Could you check a few things on this model? Use its own coordinates, in mm. A direction names the side the tool comes from. Give positions to 0.01 mm unless a question says otherwise; leave off trailing zeros. Loops run counter-clockwise (first coordinate to the right, second up) from the corner with the lowest first, then second, coordinate; pieces in that order, holes last.
1. Imagine slicing it at C-C (z = 0). List the corners of the cut face in (x, y) for me.
2. Imagine slicing it at B-B (x = -7). List the corners of the cut face in (y, z) for me.
3. Thinking about a two-plate mould opening in Z: for faces 1 (the cylindrical face through (-53.766, 14.79, -2.493)), 2 (the flat face through (-16.47, 24.2, 12.93)), 3 (the cylindrical face through (-18.221, 24.463, 4.504)), 4 (the flat face through (46, 15, -3)), which applies, +Z half, -Z half, draft (parallel to the pull), parting line (faces both ways), or undercut?
4. I need wall thicknesses on line 1 along X through (y, z) = (2.5, 5); line 2 along X through (y, z) = (25, 6.5); line 3 along X through (y, z) = (6, 10). Which ranges of each line are inside material? Lowest first, please.
5. For P1, Ø3, axis at x = -20.5, y = 14, coming from the +Z side; P2, Ø4.5, axis at y = 9.5, z = 12, coming from the -X side; P3, Ø2, axis at x = 32, y = 20, coming from the +Z side; P4, Ø14, axis at x = 137.46, z = 0, coming from the -Y side, each with a flat end and sliding along its axis, tell me the tip position at first contact or that it passes through.
6. Imagine slicing it at A-A (y = 7). List the corners of the cut face in (x, z) for me.
7. For faces 5 (the flat face through (-14.267, 22.159, 7.353)), 6 (the flat face through (14.198, 10, 13)), 7 (the flat face through (-25, 18, 3)), 8 (the flat face through (-3, 4.8, 18)), 9 (the flat face through (56, 30, 0)), which set-ups out of +Z, -Z, +X, -X, +Y, -Y let a thin tool reach every point of the face, with its end or its side?
8. Imagine slicing it at D-D (x = 84.5). List the corners of the cut face in (y, z) for me, plus the area to 3 significant figures.
```python
from build123d import *

# Parameters (mm, degrees)
SKETCH1_R           = 11.5
BOSS_EXTRUDE1_DEPTH = 30
CUT_EXTRUDE1_DEPTH  = 10
BOSS_EXTRUDE2_DEPTH = 15
SKETCH4_W           = 34
SKETCH4_H           = 2.123618691
BOSS_EXTRUDE3_DEPTH = 15
FILLET1_R           = 5
SKETCH5_R           = 10.25
CUT_EXTRUDE2_DEPTH  = 15


with BuildPart() as part:
    # Sketch1 → Boss-Extrude1 (new body)
    with BuildSketch(Plane(origin=(0, 0, 0), x_dir=(1, 0, 0), z_dir=(0, 1, 0))):
        with BuildLine():
            Line((-28.353157483, 3), (123.274320599, 3))
            ThreePointArc((123.274320599, 3), (151.960581558, 0), (123.274320599, -3))
            Line((123.274320599, -3), (-28.353157483, -3))
            ThreePointArc((-28.353157483, -3), (-57.039418442, 0), (-28.353157483, 3))
        make_face()
        with Locations(Location((-42.539418442, 0, 0), (0, 0, 270))):
            Circle(SKETCH1_R, mode=Mode.SUBTRACT)
        with Locations(Location((137.460581558, 0, 0), (0, 0, 270))):
            Circle(SKETCH1_R, mode=Mode.SUBTRACT)
    extrude(amount=BOSS_EXTRUDE1_DEPTH)

    # Sketch2 → Cut-Extrude1 (cut)
    with BuildSketch(Plane.XY.offset(3)):
        Polygon((6.198144817, 24.623618691), (-11.801855183, 24.623618691), (-16.801855183, 19.623618691), (-16.801855183, 5.123618691), (11.198144817, 5.123618691), (11.198144817, 19.623618691), align=None)
    extrude(amount=-CUT_EXTRUDE1_DEPTH, mode=Mode.SUBTRACT)

    # Sketch3 → Boss-Extrude2 (add)
    with BuildSketch(Plane.XY.offset(3)):
        Polygon((-13.044495871, 27.623618691), (7.440785504, 27.623618691), (14.198144817, 20.866259379), (14.198144817, 2.123618691), (-19.801855183, 2.123618691), (-19.801855183, 20.866259379), align=None)
        Polygon((-11.801855183, 24.623618691), (-16.801855183, 19.623618691), (-16.801855183, 5.123618691), (11.198144817, 5.123618691), (11.198144817, 19.623618691), (6.198144817, 24.623618691), align=None, mode=Mode.SUBTRACT)
    extrude(amount=BOSS_EXTRUDE2_DEPTH)

    # Sketch4 → Boss-Extrude3 (add)
    with BuildSketch(Plane.XY.offset(3)):
        with Locations((-2.801855183, 1.061809346)):
            Rectangle(SKETCH4_W, SKETCH4_H)
    extrude(amount=BOSS_EXTRUDE3_DEPTH)

    # Fillet1
    # the kernel refuses this fillet: 5 mm, written as the material it adds along each edge
    with BuildSketch(Plane(origin=(-28.640689948, 12.027424614, 3), x_dir=(-0.7071067811865481, 0.7071067811865469, 0), z_dir=(0.707106781186547, 0.7071067811865481, 0))) as fillet1_piece_1_section:
        with BuildLine():
            CenterArc((FILLET1_R, FILLET1_R), FILLET1_R, 180, 90)
            Line((0, FILLET1_R), (0, 0))
            Line((0, 0), (FILLET1_R, 0))
        make_face()
    fillet1_piece_1 = extrude(amount=34.556349186, mode=Mode.PRIVATE)
    fillet1_piece_1 = split(fillet1_piece_1, bisect_by=Plane(origin=(-28.640689948, 27.623618691, 3), z_dir=(0, -1, 0)), keep=Keep.TOP, mode=Mode.PRIVATE)
    fillet1_piece_1 = split(fillet1_piece_1, bisect_by=Plane(origin=(-19.801855183, 12.027424614, 3), z_dir=(1, 0, 0)), keep=Keep.TOP, mode=Mode.PRIVATE)
    add(fillet1_piece_1)
    with BuildSketch(Plane(origin=(-28.640689948, 12.027424614, 3), x_dir=(-0.7071067811865481, 0.7071067811865469, 0), z_dir=(0.707106781186547, 0.7071067811865481, 0))) as fillet1_piece_2_section:
        with BuildLine():
            CenterArc((FILLET1_R, FILLET1_R), FILLET1_R, 180, 90)
            Line((0, FILLET1_R), (0, 0))
            Line((0, 0), (FILLET1_R, 0))
        make_face()
    fillet1_piece_2 = extrude(amount=34.556349186, mode=Mode.PRIVATE)
    fillet1_piece_2 = split(fillet1_piece_2, bisect_by=Plane(origin=(-28.640689948, 27.623618691, 3), z_dir=(0, 1, 0)), keep=Keep.TOP, mode=Mode.PRIVATE)
    fillet1_piece_2 = split(fillet1_piece_2, bisect_by=Plane(origin=(-19.801855183, 12.027424614, 3), z_dir=(-1, 0, 0)), keep=Keep.TOP, mode=Mode.PRIVATE)
    add(fillet1_piece_2)
    with BuildSketch(Plane(origin=(-19.801855183, 0, 3), x_dir=(-1, 0, 0), z_dir=(0, 1, 0))) as fillet1_piece_3_section:
        with BuildLine():
            CenterArc((FILLET1_R, FILLET1_R), FILLET1_R, 180, 90)
            Line((0, FILLET1_R), (0, 0))
            Line((0, 0), (FILLET1_R, 0))
        make_face()
    fillet1_piece_3 = extrude(amount=33.366259379, mode=Mode.PRIVATE)
    fillet1_piece_3 = split(fillet1_piece_3, bisect_by=Plane(origin=(-30.234984873, 10.433129689, 3), z_dir=(0.7071067811865481, -0.707106781186547, 0)), keep=Keep.TOP, mode=Mode.PRIVATE)
    add(fillet1_piece_3)
    with BuildSketch(Plane(origin=(14.198144817, 33.366259379, 3), x_dir=(1, 0, 0), z_dir=(0, -1, 0))) as fillet1_piece_4_section:
        with BuildLine():
            CenterArc((FILLET1_R, FILLET1_R), FILLET1_R, 180, 90)
            Line((0, FILLET1_R), (0, 0))
            Line((0, 0), (FILLET1_R, 0))
        make_face()
    fillet1_piece_4 = extrude(amount=33.366259379, mode=Mode.PRIVATE)
    fillet1_piece_4 = split(fillet1_piece_4, bisect_by=Plane(origin=(7.948144817, 27.116259379, 3), z_dir=(-0.7071067811865476, -0.7071067811865476, 0)), keep=Keep.TOP, mode=Mode.PRIVATE)
    add(fillet1_piece_4)
    with BuildSketch(Plane(origin=(-1.398049261, 36.462453456, 3), x_dir=(0.7071067811865475, 0.7071067811865475, 0), z_dir=(0.7071067811865476, -0.7071067811865476, 0))) as fillet1_piece_5_section:
        with BuildLine():
            CenterArc((FILLET1_R, FILLET1_R), FILLET1_R, 180, 90)
            Line((0, FILLET1_R), (0, 0))
            Line((0, 0), (FILLET1_R, 0))
        make_face()
    fillet1_piece_5 = extrude(amount=34.556349186, mode=Mode.PRIVATE)
    fillet1_piece_5 = split(fillet1_piece_5, bisect_by=Plane(origin=(14.198144817, 36.462453456, 3), z_dir=(-1, 0, 0)), keep=Keep.TOP, mode=Mode.PRIVATE)
    fillet1_piece_5 = split(fillet1_piece_5, bisect_by=Plane(origin=(-1.398049261, 27.623618691, 3), z_dir=(0, -1, 0)), keep=Keep.TOP, mode=Mode.PRIVATE)
    add(fillet1_piece_5)
    with BuildSketch(Plane(origin=(-1.398049261, 36.462453456, 3), x_dir=(0.7071067811865475, 0.7071067811865475, 0), z_dir=(0.7071067811865476, -0.7071067811865476, 0))) as fillet1_piece_6_section:
        with BuildLine():
            CenterArc((FILLET1_R, FILLET1_R), FILLET1_R, 180, 90)
            Line((0, FILLET1_R), (0, 0))
            Line((0, 0), (FILLET1_R, 0))
        make_face()
    fillet1_piece_6 = extrude(amount=34.556349186, mode=Mode.PRIVATE)
    fillet1_piece_6 = split(fillet1_piece_6, bisect_by=Plane(origin=(14.198144817, 36.462453456, 3), z_dir=(1, 0, 0)), keep=Keep.TOP, mode=Mode.PRIVATE)
    fillet1_piece_6 = split(fillet1_piece_6, bisect_by=Plane(origin=(-1.398049261, 27.623618691, 3), z_dir=(0, 1, 0)), keep=Keep.TOP, mode=Mode.PRIVATE)
    add(fillet1_piece_6)
    with BuildSketch(Plane(origin=(-23.685403069, 27.623618691, 3), x_dir=(0, 1, 0), z_dir=(1, 0, 0))) as fillet1_piece_7_section:
        with BuildLine():
            CenterArc((5, 4.256362879), FILLET1_R, 180, 58.350352686)
            Line((0, 4.256362879), (0, 0))
            Line((0, 0), (2.376381309, 0))
        make_face()
    fillet1_piece_7 = extrude(amount=41.767095772, mode=Mode.PRIVATE)
    fillet1_piece_7 = split(fillet1_piece_7, bisect_by=Plane(origin=(-8.122308783, 43.186712978, 3), z_dir=(-0.7071067811865476, -0.7071067811865476, 0)), keep=Keep.TOP, mode=Mode.PRIVATE)
    fillet1_piece_7 = split(fillet1_piece_7, bisect_by=Plane(origin=(-18.36494947, 22.303165092, 3), z_dir=(0.7071067811865481, -0.707106781186547, 0)), keep=Keep.TOP, mode=Mode.PRIVATE)
    add(fillet1_piece_7)
    with BuildSketch(Plane(origin=(-19.801855183, 0, 3), x_dir=(-1, 0, 0), z_dir=(0, 1, 0))) as fillet1_piece_8a_section:
        with BuildLine():
            CenterArc((FILLET1_R, FILLET1_R), FILLET1_R, 180, 90)
            Line((0, FILLET1_R), (0, 0))
            Line((0, 0), (FILLET1_R, 0))
        make_face()
    fillet1_piece_8a = extrude(amount=33.366259379, mode=Mode.PRIVATE)
    fillet1_piece_8a = split(fillet1_piece_8a, bisect_by=Plane(origin=(-30.234984873, 10.433129689, 3), z_dir=(-0.7071067811865481, 0.707106781186547, 0)), keep=Keep.TOP, mode=Mode.PRIVATE)
    fillet1_piece_8a = split(fillet1_piece_8a, bisect_by=Plane(origin=(-19.801855183, 30, 3), z_dir=(0, -1, 0)), keep=Keep.TOP, mode=Mode.PRIVATE)
    with BuildSketch(Plane(origin=(-28.640689948, 12.027424614, 3), x_dir=(-0.7071067811865481, 0.7071067811865469, 0), z_dir=(0.707106781186547, 0.7071067811865481, 0))) as fillet1_piece_8b_section:
        with BuildLine():
            CenterArc((FILLET1_R, FILLET1_R), FILLET1_R, 180, 90)
            Line((0, FILLET1_R), (0, 0))
            Line((0, 0), (FILLET1_R, 0))
        make_face()
    fillet1_piece_8b = extrude(amount=34.556349186, mode=Mode.PRIVATE)
    fillet1_piece_8b = split(fillet1_piece_8b, bisect_by=Plane(origin=(-19.801855183, 12.027424614, 3), z_dir=(-1, 0, 0)), keep=Keep.TOP, mode=Mode.PRIVATE)
    fillet1_piece_8b = fillet1_piece_8b - Plane(origin=(-42.539418442, 12.027424614, 0), x_dir=(0.9783628247662832, 0, 0.20689655172413826), z_dir=(0, -1, 0)) * Cylinder(14.5, 90, mode=Mode.PRIVATE)
    fillet1_piece_8 = fillet1_piece_8a & fillet1_piece_8b
    add(fillet1_piece_8)
    with BuildSketch(Plane(origin=(-28.640689948, 12.027424614, 3), x_dir=(-0.7071067811865481, 0.7071067811865469, 0), z_dir=(0.707106781186547, 0.7071067811865481, 0))) as fillet1_piece_9a_section:
        with BuildLine():
            CenterArc((FILLET1_R, FILLET1_R), FILLET1_R, 180, 90)
            Line((0, FILLET1_R), (0, 0))
            Line((0, 0), (FILLET1_R, 0))
        make_face()
    fillet1_piece_9a = extrude(amount=34.556349186, mode=Mode.PRIVATE)
    fillet1_piece_9a = split(fillet1_piece_9a, bisect_by=Plane(origin=(-28.640689948, 27.623618691, 3), z_dir=(0, 1, 0)), keep=Keep.TOP, mode=Mode.PRIVATE)
    fillet1_piece_9a = split(fillet1_piece_9a, bisect_by=Plane(origin=(-28.640689948, 30, 3), z_dir=(0, -1, 0)), keep=Keep.TOP, mode=Mode.PRIVATE)
    with BuildSketch(Plane(origin=(-23.685403069, 27.623618691, 3), x_dir=(0, 1, 0), z_dir=(1, 0, 0))) as fillet1_piece_9b_section:
        with BuildLine():
            CenterArc((5, 4.256362879), FILLET1_R, 180, 58.350352686)
            Line((0, 4.256362879), (0, 0))
            Line((0, 0), (2.376381309, 0))
        make_face()
    fillet1_piece_9b = extrude(amount=41.767095772, mode=Mode.PRIVATE)
    fillet1_piece_9b = split(fillet1_piece_9b, bisect_by=Plane(origin=(-18.36494947, 22.303165092, 3), z_dir=(-0.7071067811865481, 0.707106781186547, 0)), keep=Keep.TOP, mode=Mode.PRIVATE)
    fillet1_piece_9 = fillet1_piece_9a & fillet1_piece_9b
    add(fillet1_piece_9)
    with BuildSketch(Plane(origin=(-1.398049261, 36.462453456, 3), x_dir=(0.7071067811865475, 0.7071067811865475, 0), z_dir=(0.7071067811865476, -0.7071067811865476, 0))) as fillet1_piece_10a_section:
        with BuildLine():
            CenterArc((FILLET1_R, FILLET1_R), FILLET1_R, 180, 90)
            Line((0, FILLET1_R), (0, 0))
            Line((0, 0), (FILLET1_R, 0))
        make_face()
    fillet1_piece_10a = extrude(amount=34.556349186, mode=Mode.PRIVATE)
    fillet1_piece_10a = split(fillet1_piece_10a, bisect_by=Plane(origin=(14.198144817, 36.462453456, 3), z_dir=(1, 0, 0)), keep=Keep.TOP, mode=Mode.PRIVATE)
    with BuildSketch(Plane(origin=(14.198144817, 33.366259379, 3), x_dir=(1, 0, 0), z_dir=(0, -1, 0))) as fillet1_piece_10b_section:
        with BuildLine():
            CenterArc((FILLET1_R, FILLET1_R), FILLET1_R, 180, 90)
            Line((0, FILLET1_R), (0, 0))
            Line((0, 0), (FILLET1_R, 0))
        make_face()
    fillet1_piece_10b = extrude(amount=33.366259379, mode=Mode.PRIVATE)
    fillet1_piece_10b = split(fillet1_piece_10b, bisect_by=Plane(origin=(7.948144817, 27.116259379, 3), z_dir=(0.7071067811865476, 0.7071067811865476, 0)), keep=Keep.TOP, mode=Mode.PRIVATE)
    fillet1_piece_10b = split(fillet1_piece_10b, bisect_by=Plane(origin=(14.198144817, 30, 3), z_dir=(0, -1, 0)), keep=Keep.TOP, mode=Mode.PRIVATE)
    fillet1_piece_10 = fillet1_piece_10a & fillet1_piece_10b
    add(fillet1_piece_10)
    with BuildSketch(Plane(origin=(-23.685403069, 27.623618691, 3), x_dir=(0, 1, 0), z_dir=(1, 0, 0))) as fillet1_piece_11a_section:
        with BuildLine():
            CenterArc((5, 4.256362879), FILLET1_R, 180, 58.350352686)
            Line((0, 4.256362879), (0, 0))
            Line((0, 0), (2.376381309, 0))
        make_face()
    fillet1_piece_11a = extrude(amount=41.767095772, mode=Mode.PRIVATE)
    fillet1_piece_11a = split(fillet1_piece_11a, bisect_by=Plane(origin=(-8.122308783, 43.186712978, 3), z_dir=(0.7071067811865476, 0.7071067811865476, 0)), keep=Keep.TOP, mode=Mode.PRIVATE)
    with BuildSketch(Plane(origin=(-1.398049261, 36.462453456, 3), x_dir=(0.7071067811865475, 0.7071067811865475, 0), z_dir=(0.7071067811865476, -0.7071067811865476, 0))) as fillet1_piece_11b_section:
        with BuildLine():
            CenterArc((FILLET1_R, FILLET1_R), FILLET1_R, 180, 90)
            Line((0, FILLET1_R), (0, 0))
            Line((0, 0), (FILLET1_R, 0))
        make_face()
    fillet1_piece_11b = extrude(amount=34.556349186, mode=Mode.PRIVATE)
    fillet1_piece_11b = split(fillet1_piece_11b, bisect_by=Plane(origin=(-1.398049261, 27.623618691, 3), z_dir=(0, 1, 0)), keep=Keep.TOP, mode=Mode.PRIVATE)
    fillet1_piece_11b = split(fillet1_piece_11b, bisect_by=Plane(origin=(-1.398049261, 30, 3), z_dir=(0, -1, 0)), keep=Keep.TOP, mode=Mode.PRIVATE)
    fillet1_piece_11 = fillet1_piece_11a & fillet1_piece_11b
    add(fillet1_piece_11)

    # Sketch5 → Cut-Extrude2 (cut)
    with BuildSketch(Plane(origin=(0, 0, -3), x_dir=(-1, 0, 0), z_dir=(0, 0, -1))):
        with Locations((-103.805830626, 15.139955724)):
            Circle(SKETCH5_R)
    extrude(amount=-CUT_EXTRUDE2_DEPTH, mode=Mode.SUBTRACT)


solid = part.part
```
Derived:
1. outline: (-57.04, 0) - (-54.04, 0) - (-54.04, 30) - (-57.04, 30) - close; (-31.04, 0) - (125.96, 0) - (125.96, 30) - (-31.04, 30) - close; (148.96, 0) - (151.96, 0) - (151.96, 30) - (148.96, 30) - close; hole (-16.8, 5.12) - (11.2, 5.12) - (11.2, 19.62) - (6.2, 24.62) - (-11.8, 24.62) - (-16.8, 19.62) - close; hole circle Ø20.5 at (103.81, 15.14)
2. outline: (0, -3) - (5.12, -3) - (5.12, 18) - (0, 18) - close; (24.62, -3) - (30, -3) - (30, 3) arc R5 cw to (27.62, 7.26) - (27.62, 18) - (24.62, 18) - close
3. face 1: undercut
3. face 2: draft
3. face 3: +Z half
3. face 4: -Z half
4. line 1: x = -56.15 to -52.9, -32.18 to -28.93, -20.8 to 15.2, 123.85 to 127.1, 147.82 to 151.07
4. line 2: x = -55.5 to -52.03, -33.05 to -29.58, -15.99 to 10.39, 124.5 to 127.97, 146.95 to 150.42
4. line 3: x = -53.04 to -48.22, -36.86 to -32.04, -19.8 to -16.8, 11.2 to 14.2, 126.96 to 131.78, 143.14 to 147.96
5. P1: stops at z = 18
5. P2: stops at x = -53.27
5. P3: stops at z = 3
5. P4: passes through
6. outline: (-28.35, -3) - (-16.8, -3) - (-16.8, 18) - (-19.8, 18) - (-19.8, 8) arc R5 cw to (-24.8, 3) - (-28.35, 3) arc R14.5 ccw (long way) to start; (11.2, -3) - (97.58, -3) - (97.58, 3) - (19.2, 3) arc R5 cw to (14.2, 8) - (14.2, 18) - (11.2, 18) - close; (110.04, -3) - (123.27, -3) arc R14.5 ccw (long way) to (123.27, 3) - (110.04, 3) - close; hole circle Ø23 at (-42.54, 0); hole circle Ø23 at (137.46, 0)
7. face 5: +Z, -Z
7. face 6: +Z, +Y, -Y
7. face 7: +Z, +Y
7. face 8: +Z, +X, -X, +Y, -Y
7. face 9: +Z, -Z, +X, -X, +Y
8. outline: (0, -3) - (30, -3) - (30, 3) - (0, 3) - close
8. area: 180 mm2
